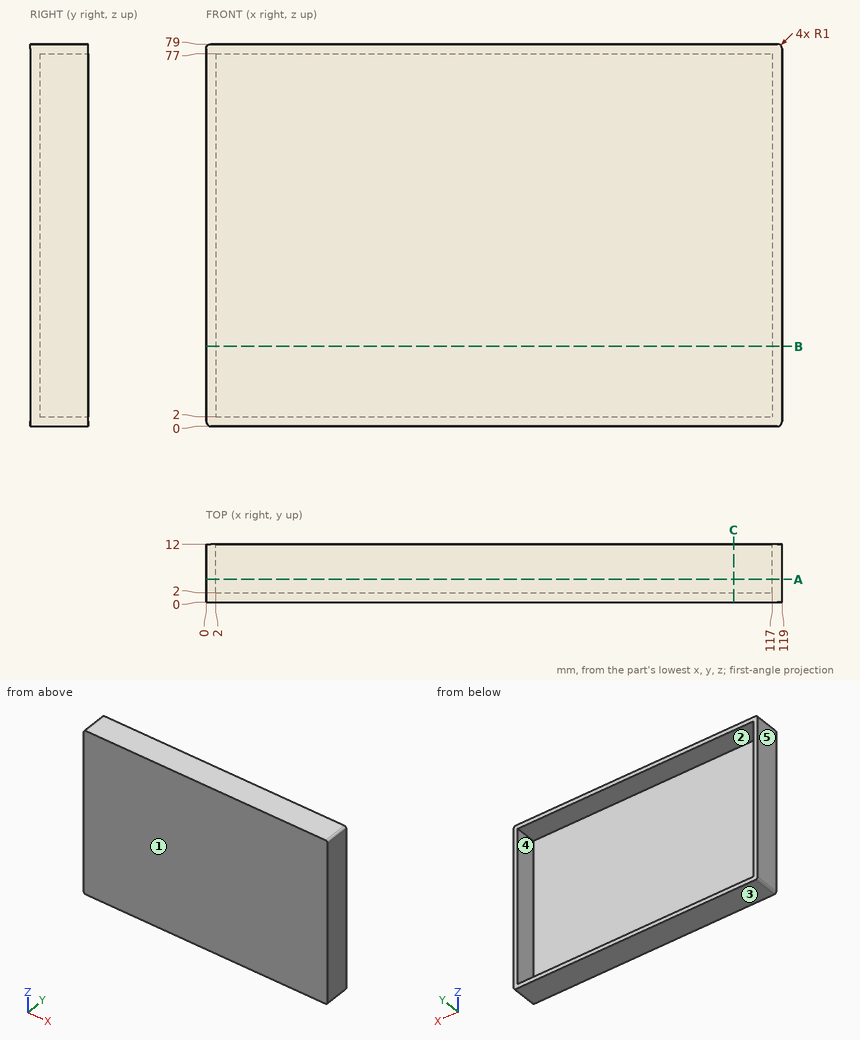
Geometry check sheet. Reference: drawing and pictorial views, mm from the part's lowest x, y, z. A direction names the side the tool comes from. Round coordinates to 2 decimals unless told otherwise and drop trailing zeros. Write each loop counter-clockwise with the first axis right and the second up, starting at its lowest first coordinate (ties: lowest second). Pieces come first, ordered by that corner, then holes.
(1) Depth check by flat-ended pin: pin 1 Ø10 at (x, z) = (79, 16.5) entering from +Y. Enter the tip coordinate at first touch or a pass-through.
Returned:
pin 1: stops at y = 2
(2) Mould release check, pull along Z, two halves, no side actions. Record for the marked faces 1, 2 and 3: pulls with the +Z half, pulls with the -Z half, needs draft (parallel to the pull), parting line crosses it, or undercut.
Returned:
face 1: needs draft
face 2: undercut
face 3: pulls with the -Z half
(3) Section check B-B (z = 16.5). Enter the section's corners in (x, y), plus the area to 3 significant figures.
Returned:
outline: (0, 0) - (119, 0) - (119, 12) - (117, 12) - (117, 2) - (2, 2) - (2, 12) - (0, 12) - close
area: 278 mm2
(4) Material ranges on line 1 (X direction, y = 10, z = 73); line 2 (Z direction, x = 89, y = 9.75); line 3 (Y direction, x = 59, z = 76.5), recorded low to high.
Returned:
line 1: x = 0 to 2, 117 to 119
line 2: z = 0 to 2, 77 to 79
line 3: y = 0 to 2
(5) Section check C-C (x = 109). Enter the section's corners in (y, z), plus the area to 3 significant figures.
Returned:
outline: (0, 0) - (12, 0) - (12, 2) - (2, 2) - (2, 77) - (12, 77) - (12, 79) - (0, 79) - close
area: 198 mm2
(6) Access from +Z, -Z, +X, -X, +Y, -Y to the whole of each face (thin tool, end or side, straight path). Record for the marked faces 4 and 5.
Returned:
face 4: +Y
face 5: +Z, -Z, -X, +Y, -Y
(7) Section check A-A (y = 4.75). Enter the section's corners in (x, z).
Returned:
outline: (0, 1) arc R1 ccw to (1, 0) - (118, 0) arc R1 ccw to (119, 1) - (119, 78) arc R1 ccw to (118, 79) - (1, 79) arc R1 ccw to (0, 78) - close; hole (2, 2) - (117, 2) - (117, 77) - (2, 77) - close
